CAD build for the part. Positions are in the model's coordinates, mm. Coordinates: 2 decimals unless noted, no trailing zeros. Write each loop counter-clockwise with the first axis right and the second up, starting at its lowest first coordinate (ties: lowest second). Pieces come first, ordered by that corner, then holes. Notation, with made-up numbers: M 20,69.5 L 24,69.5 A25 cw 24,88.5 Z; hole C 72.5,-5.75 d1. An arc over 180 degrees is marked long. Put each result on its own line as item: value. Start each with the question number.
```python
from build123d import *

# Parameters (mm, degrees)
BOSS_EXTRUDE1_DEPTH = 67
SKETCH2_R           = 3.2
CUT_EXTRUDE1_DEPTH  = 73.467233975


with BuildPart() as part:
    # Sketch1 → Boss-Extrude1 (new body)
    with BuildSketch(Plane(origin=(0, 0, 0), x_dir=(0, 0, -1), z_dir=(1, 0, 0))):
        with BuildLine():
            Line((-23.5, -58.2), (23.5, -58.2))
            Line((23.5, -58.2), (23.5, -68.797092962))
            ThreePointArc((23.5, -68.797092962), (0, -72.7), (-23.5, -68.797092962))
            Line((-23.5, -68.797092962), (-23.5, -58.2))
        make_face()
    extrude(amount=BOSS_EXTRUDE1_DEPTH)

    # Sketch2 → Cut-Extrude1 (cut, through all)
    with BuildSketch(Plane(origin=(0, -58.2, 0), x_dir=(1, 0, 0), z_dir=(0, 1, 0))):
        with Locations(Location((23, 0, 0), (0, 0, 270))):
            Circle(SKETCH2_R)
    extrude(amount=-CUT_EXTRUDE1_DEPTH, mode=Mode.SUBTRACT)


solid = part.part
```
(1) Slice it at C-C, the plane z = -9.5. Write the cut outline in (x, y), then the cut area to 3 significant figures.
(2) Slice it at A-A, the plane z = 0. Write the cut outline in (x, y).
(3) Drop flat-ended pins along their axis: pin 1 (1 mm diameter, centred on x = 15, z = 2, fed in from -Y); pin 2 (1 mm diameter, centred on x = 54, z = -15, fed in from -Y); pin 3 (8 mm diameter, centred on x = 25.5, z = 11.5, fed in from -Y). Give the stop position or say it passes through.
(4) Slice it at B-B, the plane x = 23. Write the cut outline in (y, z).
(5) Drill centre lines: line 1 (Z direction, x = 23, y = -61.5); line 2 (X direction, y = -63, z = 0); line 3 (Z direction, x = 22, y = -67.5). Where is each one in solid material? Low to high. Write a range as [from, to].
(6) Two-plate mould, pull along X, no slides. Class faces 1 (the face through (0, -65, 0)), 2 (the face through (33, -64, 23.5)), 3 (the face through (67, -65, 0)), 4 (the face through (26.173, -65.35, -0.417)): +X half, -X half, draft (parallel to the pull), parting line (faces both ways), or undercut.
Result set:
1. outline: M 0,-72.08 L 67,-72.08 L 67,-58.2 L 0,-58.2 Z
1. area: 930 mm^2
2. outline: M 0,-72.7 L 19.8,-72.7 L 19.8,-58.2 L 0,-58.2 Z; M 26.2,-72.7 L 67,-72.7 L 67,-58.2 L 26.2,-58.2 Z
3. pin 1: stops at y = -72.68
3. pin 2: stops at y = -71.24
3. pin 3: stops at y = -72.31
4. outline: M -72.63,-3.2 A72.7 ccw -68.8,-23.5 L -58.2,-23.5 L -58.2,-3.2 Z; M -72.63,3.2 L -58.2,3.2 L -58.2,23.5 L -68.8,23.5 A72.7 ccw Z
5. line 1: z = [-23.5, -3.2], [3.2, 23.5]
5. line 2: x = [0, 19.8], [26.2, 67]
5. line 3: z = [-23.5, -3.04], [3.04, 23.5]
6. face 1: -X half
6. face 2: draft
6. face 3: +X half
6. face 4: undercut
